For this review, take the finished solid that the model builds, in its own axes (mm). A direction names the side the tool comes from. Give positions to 0.01 mm unless a question says otherwise; leave off trailing zeros. Order: outer loops, then holes, each group sorted by start corner. A loop starts at its lowest first (then second) coordinate and runs counter-clockwise, first axis right, second up. Notation, with made-up numbers: (45, -31.5) - (102, -31.5) arc R28 cw to (102, -13.5) - close; hole circle Ø9 at (57.25, 46). An arc over 180 degrees is marked (long way). Use a Markdown table: item, result. Add a question column.
1) Wall thickness on L1, parallel to Z at x = 1.3, y = 19.9 (3 decimals); L2, parallel to Z at x = 0.75, y = 19.85 (3 decimals); L3, parallel to Y at x = 2.3, z = 3.3 (3 decimals): over which ranges is each line inside the solid? List them lowest first.
2) Clearance check with flat-ended pins moving along their axes: P1, Ø1.5, axis at y = 20.5, z = 7.5, coming from the -X side; P2, Ø1.5, axis at y = 20, z = 3.3, coming from the -X side; P3, Ø0.5, axis at x = 1.5, z = 9, coming from the -Y side. State where each tip first meets the part, or that it passes through.
3) Machinability: for faces 1 (the face through (1.43, 19.507, 6.14)), 2 (the face through (0, 20, 2)), 3 (the face through (0.5, 21, 7)), which of the approach directions +Z, -Z, +X, -X, +Y, -Y give a long, thin tool a straight path to every point of the face, cutting with its end or side? Answer none if there is none.
4) We need section D-D on z = 3.3. Write out the cut boundary in (x, y) (3 decimals), then the cut area to 4 significant figures.
5) We need section A-A on z = 0. Write out the cut boundary in (x, y) (3 decimals).
6) Mouldability with a two-part tool opening along Z and no side actions: class faces 4 (the face through (1, 20, 9.425)), 5 (the face through (2.1, 21, 8)), 6 (the face through (1.43, 20.82, -0.43)) as released by +Z, released by -Z, zero draft, split by the parting line, or undercut.
7) We need section B-B on x = 0.7. Write out the cut boundary in (y, z) (3 decimals), then the cut area to 3 significant figures.
```python
from build123d import *

# Parameters (mm, degrees)
SKETCH_1_W          = 11.5
SKETCH_1_H          = 3
SKETCH_1_R          = 0.925
SKETCH_1_R_2        = 0.825
SKETCH_1_R_3        = 0.8
EXTRUDE_1_DEPTH     = 2.9
CUT_EXTRUDE_1_DEPTH = 11.06184004
SKETCH_2_W          = 0.5
SKETCH_2_H          = 4.4
SKETCH_2_W_2        = 0.8
SKETCH_2_H_2        = 3.4
CUT_EXTRUDE_2_DEPTH = 11.3073093
FILLET_2_R          = 1
FILLET_3_R          = 0.5
SKETCH_3_W          = 47.443490455
SKETCH_3_H          = 29.152776371
CUT_EXTRUDE_3_DEPTH = 16.531922772


with BuildPart() as part:
    # 草图1 → 凸台-拉伸1 (new body)
    with BuildSketch(Plane(origin=(0, 0, 0), x_dir=(0, 0, -1), z_dir=(1, 0, 0))):
        with Locations((-3.675, -0.5)):
            Rectangle(SKETCH_1_W, SKETCH_1_H)
        Circle(SKETCH_1_R, mode=Mode.SUBTRACT)
        with Locations((-3.3, 0)):
            Circle(SKETCH_1_R_2, mode=Mode.SUBTRACT)
        with Locations((-8.025, 0)):
            Circle(SKETCH_1_R_3, mode=Mode.SUBTRACT)
    extrude(amount=EXTRUDE_1_DEPTH)

    # 草图1<11> → 切除-拉伸1 (cut, through all)
    with BuildSketch(Plane(origin=(0, 0, 0), x_dir=(0, 0, -1), z_dir=(1, 0, 0))):
        with BuildLine():
            Line((-8.825, 0.5), (-8.825, 0))
            ThreePointArc((-8.825, 0), (-8.025, 0.8), (-7.225, 0))
            Line((-7.225, 0), (-5.025, 1))
            Line((-5.025, 1), (-9.425, 1))
            Line((-9.425, 1), (-9.425, 0.5))
            Line((-9.425, 0.5), (-8.825, 0.5))
        make_face()
    extrude(amount=CUT_EXTRUDE_1_DEPTH, mode=Mode.SUBTRACT)

    # 草图2 → 切除-拉伸2 (cut, through all)
    with BuildSketch(Plane.XZ.offset(2)):
        with Locations((0.25, 7.225)):
            Rectangle(SKETCH_2_W, SKETCH_2_H)
        with Locations((2.5, 7.725)):
            Rectangle(SKETCH_2_W_2, SKETCH_2_H_2)
    extrude(amount=-CUT_EXTRUDE_2_DEPTH, mode=Mode.SUBTRACT)

    # 圆角2
    fillet_2_edges = [part.edges().sort_by_distance(p)[0] for p in [
        (1.45, -2, -2.075),
        (1.3, -2, 9.425),
    ]]
    fillet(fillet_2_edges, radius=FILLET_2_R)

    # 圆角3
    fillet_3_edges = [part.edges().sort_by_distance(p)[0] for p in [
        (2.9, -0.727272727, 6.025),
        (0.5, -0.5, 5.025),
    ]]
    fillet(fillet_3_edges, radius=FILLET_3_R - 0.0001)  # a hair under: the kernel refuses the full size


with BuildPart() as body_2:
    # 镜向1: mirrored copy
    add(part.part.mirror(Plane.ZX.offset(10)))


with BuildPart() as part_1:
    add(part.part)

    # 草图3 → 切除-拉伸3 (cut, through all)
    with BuildSketch(Plane(origin=(0, 10, 0), x_dir=(1, 0, 0), z_dir=(0, 1, 0))):
        with Locations((5.281098752, -2.215269705)):
            Rectangle(SKETCH_3_W, SKETCH_3_H)
    extrude(amount=-CUT_EXTRUDE_3_DEPTH, mode=Mode.SUBTRACT)


solid = body_2.part
```
Checked values:
| question | item | result |
|---|---|---|
| 1 | L1 | -2.075 to -0.92, 0.92 to 2.481, 4.119 to 7.005, 8.825 to 9.425 |
| 1 | L2 | -2.075 to -0.913, 0.913 to 2.489, 4.111 to 6.895, 8.825 to 9.425 |
| 1 | L3 | 19 to 19.175, 20.825 to 22 |
| 2 | P1 | x = 0.5 |
| 2 | P2 | through |
| 2 | P3 | y = 19.5 |
| 3 | face 1 | +X, -X, -Y |
| 3 | face 2 | +Z, -Z, -X, +Y, -Y |
| 3 | face 3 | +Z, -X, +Y, -Y |
| 4 | outline | (0, 19) - (2.9, 19) - (2.9, 19.175) - (0, 19.175) - close; (0, 20.825) - (2.9, 20.825) - (2.9, 22) - (0, 22) - close |
| 4 | area | 3.915 mm² |
| 5 | outline | (0, 19) - (2.9, 19) - (2.9, 19.075) - (0, 19.075) - close; (0, 20.925) - (2.9, 20.925) - (2.9, 22) - (0, 22) - close |
| 6 | face 4 | released by +Z |
| 6 | face 5 | zero draft |
| 6 | face 6 | undercut |
| 7 | outline | (19, -2.075) - (21, -2.075) arc R1 ccw to (22, -1.075) - (22, 8.425) arc R1 ccw to (21, 9.425) - (19.5, 9.425) - (19.5, 8.825) - (20, 8.825) arc R0.8 cw to (20, 7.225) - (19, 5.025) - close; hole circle Ø1.85 at (20, 0); hole circle Ø1.65 at (20, 3.3) |
| 7 | area | 25.2 mm² |
